from build123d import *

# Parameters (mm, degrees)
SKETCH1_R                = 36
BOSS_EXTRUDE1_DEPTH      = 18
SKETCH2_W                = 36
SKETCH2_H                = 36
BOSS_EXTRUDE2_DEPTH      = 109
SKETCH3_R                = 15
BOSS_EXTRUDE3_DEPTH      = 20
SKETCH4_R                = 30
BOSS_EXTRUDE4_DEPTH      = 40
CUT_EXTRUDE1_DEPTH       = 139.351002938
CUT_EXTRUDE1_DEPTH_BACK  = 139.351002938
HOLE1_D                  = 30
CUT_EXTRUDE2_START       = -60
CUT_EXTRUDE2_DEPTH       = 244.926615935
FILLET1_R                = 5
CIRPATTERN1_COUNT        = 4
FILLET1_OF_CIRPATTERN1_R = 5


with BuildPart() as part:
    # Sketch1 → Boss-Extrude1 (new, symmetric)
    with BuildSketch(Plane(origin=(0, 0, 0), x_dir=(0, 0, -1), z_dir=(1, 0, 0))):
        Circle(SKETCH1_R)
    extrude(amount=BOSS_EXTRUDE1_DEPTH, both=True)

    # Sketch2 → Boss-Extrude2 (add)
    with BuildSketch(Plane.XY):
        Rectangle(SKETCH2_W, SKETCH2_H)
    extrude(amount=BOSS_EXTRUDE2_DEPTH)

    # Sketch3 → Boss-Extrude3 (add)
    with BuildSketch(Plane.XY.offset(109)):
        Circle(SKETCH3_R)
    extrude(amount=BOSS_EXTRUDE3_DEPTH)

    # Sketch4 → Boss-Extrude4 (add, symmetric)
    with BuildSketch(Plane(origin=(0, 0, 0), x_dir=(1, 0, 0), z_dir=(0, 1, 0))):
        with Locations(Location((0, 38, 0), (0, 0, 270))):
            Circle(SKETCH4_R)
    extrude(amount=BOSS_EXTRUDE4_DEPTH, both=True)

    # Sketch5 → Cut-Extrude1 (cut, two sides: drawn at the far end of the back side and taken through both)
    with BuildSketch(Plane(origin=(0, 0, 0), x_dir=(0, 0, -1), z_dir=(1, 0, 0)).offset(-CUT_EXTRUDE1_DEPTH_BACK)):
        with BuildLine():
            Line((0, 18), (68, 18))
            Line((68, 18), (68, -18))
            Line((68, -18), (0, -18))
            ThreePointArc((0, -18), (-18, 0), (0, 18))
        make_face()
    extrude(amount=CUT_EXTRUDE1_DEPTH + CUT_EXTRUDE1_DEPTH_BACK, mode=Mode.SUBTRACT)

    # Hole1 (through all)
    with Locations(Plane(origin=(0, 40, 0), x_dir=(1, 0, 0), z_dir=(0, 1, 0))):
        with Locations((0, 38)):
            Hole(HOLE1_D / 2)

    # Sketch8 → Cut-Extrude2 (cut)
    with BuildSketch(Plane.XY.offset(109).offset(CUT_EXTRUDE2_START)):
        with BuildLine():
            Line((13, 18), (18, 18))
            Line((18, 18), (18, 13))
            ThreePointArc((18, 13), (14.464466094, 14.464466094), (13, 18))
        make_face()
    cut_extrude2 = extrude(amount=CUT_EXTRUDE2_DEPTH, mode=Mode.SUBTRACT)

    # Fillet1
    fillet1_edges = [part.edges().sort_by_distance(p)[0] for p in [
        (14.464466094, 14.464466094, 49),
    ]]
    fillet(fillet1_edges, radius=FILLET1_R - 0.0001)  # a hair under: the kernel refuses the full size

    # CirPattern1: Cut-Extrude2 ×4 about axis
    cirpattern1_axis = Axis((0, 0, 0), (0, 0, 1))
    for i in range(1, CIRPATTERN1_COUNT):
        add(cut_extrude2.rotate(cirpattern1_axis, i * 360 / CIRPATTERN1_COUNT), mode=Mode.SUBTRACT)

    # Fillet1 of CirPattern1
    fillet1_of_cirpattern1_edges = [part.edges().sort_by_distance(p)[0] for p in [
        (-14.464466094, 14.464466094, 49),
        (-14.464466094, -14.464466094, 49),
        (14.464466094, -14.464466094, 49),
    ]]
    fillet(fillet1_of_cirpattern1_edges, radius=FILLET1_OF_CIRPATTERN1_R - 0.0001)  # a hair under: the kernel refuses the full size


solid = part.part
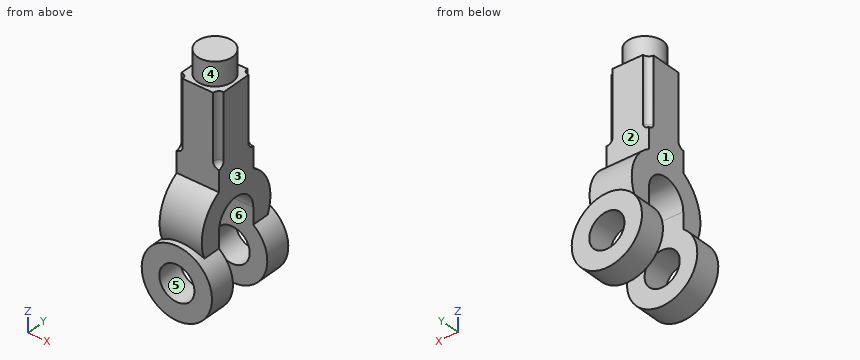
Here's how the part is built. I have some questions about the finished solid (model axes, mm). Face numbers are marked on the shaded views. A direction names the side the tool comes from. Round coordinates to 2 decimals unless told otherwise and drop trailing zeros. Order: outer loops, then holes, each group sorted by start corner. A loop starts at its lowest first (then second) coordinate and runs counter-clockwise, first axis right, second up. Notation, with made-up numbers: M 71,-36.5 L 82,-36.5 A28 cw 82,-9.5 Z; hole C 54,28 d4. An arc over 180 degrees is marked long. Return JSON: item names as keys, results as strings. Group by question number.
1. If we section it at C-C on x = 2: List the corners of the cut face in (y, z) for me, then the cut area to 3 significant figures.
2. If we section it at D-D on x = 21.5: List the corners of the cut face in (y, z) for me.
3. If we section it at B-B on y = 0: List the corners of the cut face in (x, z) for me, then the cut area to 3 significant figures.
4. Please list where these lines run through material, in increasing order: probe 1 along Y at (x, z) = (6, -22.5); probe 2 along Y at (x, z) = (10.5, 93.5); probe 3 along Y at (x, z) = (-17.5, 74.5).
5. If we section it at A-A on z = -38: List the corners of the cut face in (x, y) for me.
6. On a 3-axis mill with a long thin cutter (end or side, diameter ignored), from which of +Z, -Z, +X, -X, +Y, -Y can I reach the whole of each face in a straight line? I mean the marked faces 1, 2 and 3. Say none if no direction works.
7. I'm going to push flat-ended pins straight in: pin 1 Ø1.5 at (y, z) = (-27, -27.5) entering from +X; pin 2 Ø4 at (x, y) = (-24, -22) entering from +Z; pin 3 Ø2 at (y, z) = (16.5, 76) entering from -X. Where does each tip first touch, or does it pass through?
8. If we mould it in two halves opening along Y, with no side actions, what happens to the marked faces 4, 5 and 6? For each: pulls with the +Y half, pulls with the -Y half, needs draft (parallel to the pull), parting line crosses it, or undercut.
Reply:
{
 "1": {"outline": "M -40,-67.93 L -18,-67.93 L -18,-52.87 L -40,-52.87 Z; M -40,-23.13 L -18,-23.13 L -18,0 A18 cw 18,0 L 18,-23.13 L 40,-23.13 L 40,-8.07 L 35.08,-8.07 A36 ccw 18,31.18 L 18,109 L 14.87,109 L 14.87,129 L -14.87,129 L -14.87,109 L -18,109 L -18,31.18 A36 ccw -35.08,-8.07 L -40,-8.07 Z; M 18,-67.93 L 40,-67.93 L 40,-52.87 L 18,-52.87 Z", "area": "6,420 mm^2"},
 "2": {"outline": "M -40,-58.92 L -18,-58.92 L -18,-17.08 L -40,-17.08 Z; M 18,-58.92 L 40,-58.92 L 40,-17.08 L 18,-17.08 Z"},
 "3": {"outline": "M -18,18 L 18,18 L 18,109 L 15,109 L 15,129 L -15,129 L -15,109 L -18,109 Z", "area": "3,880 mm^2"},
 "4": {"probe 1": "-40 to -18, 18 to 40", "probe 2": "-18 to 18", "probe 3": "-13.03 to 13.03"},
 "5": {"outline": "M -30,-40 L -15,-40 L -15,-18 L -30,-18 Z; M -30,18 L -15,18 L -15,40 L -30,40 Z; M 15,-40 L 30,-40 L 30,-18 L 15,-18 Z; M 15,18 L 30,18 L 30,40 L 15,40 Z"},
 "6": {"face 1": "+Z, -X, +Y, -Y", "face 2": "+Z, +X, -X, +Y", "face 3": "+Z, +X, +Y, -Y"},
 "7": {"pin 1": "x = 28.37", "pin 2": "z = -17.6", "pin 3": "x = -13.67"},
 "8": {"face 4": "parting line crosses it", "face 5": "needs draft", "face 6": "undercut"}
}
